For this review, take the finished solid that the model builds, in its own axes (mm). Give positions to 0.01 mm unless a question says otherwise; leave off trailing zeros. Loops run counter-clockwise (first coordinate to the right, second up) from the corner with the lowest first, then second, coordinate; pieces in that order, holes last.
```python
from build123d import *

# Parameters (mm, degrees)
SKETCH_1_R      = 80
SKETCH_1_R_2    = 4
SKETCH_1_R_3    = 1.02
SKETCH_1_R_4    = 6.269952148
EXTRUDE_1_DEPTH = 3


with BuildPart() as part:
    # ｽｹｯﾁ1 → ﾎﾞｽ - 押し出し1 (new body)
    with BuildSketch(Plane(origin=(0, 0, 0), x_dir=(0, 0, -1), z_dir=(1, 0, 0))):
        Circle(SKETCH_1_R)
        Circle(SKETCH_1_R_2, mode=Mode.SUBTRACT)
        with Locations((4.949747468, 4.949747468)):
            Circle(SKETCH_1_R_3, mode=Mode.SUBTRACT)
        with Locations((7, 0)):
            Circle(SKETCH_1_R_3, mode=Mode.SUBTRACT)
        with Locations((4.949747468, -4.949747468)):
            Circle(SKETCH_1_R_3, mode=Mode.SUBTRACT)
        with Locations((0, -7)):
            Circle(SKETCH_1_R_3, mode=Mode.SUBTRACT)
        with Locations((-4.949747468, -4.949747468)):
            Circle(SKETCH_1_R_3, mode=Mode.SUBTRACT)
        with Locations((-7, 0)):
            Circle(SKETCH_1_R_3, mode=Mode.SUBTRACT)
        with Locations((-4.949747468, 4.949747468)):
            Circle(SKETCH_1_R_3, mode=Mode.SUBTRACT)
        with Locations((0, 7)):
            Circle(SKETCH_1_R_3, mode=Mode.SUBTRACT)
        with Locations((-38, 0)):
            Circle(SKETCH_1_R_4, mode=Mode.SUBTRACT)
        with BuildLine():
            Line((-30.755353243, 42.837057437), (35.175005572, 42.837057437))
            ThreePointArc((35.175005572, 42.837057437), (36.589219135, 43.422843874), (37.175005572, 44.837057437))
            Line((37.175005572, 44.837057437), (37.175005572, 45.489077015))
            ThreePointArc((37.175005572, 45.489077015), (36.589219135, 46.903290577), (35.175005572, 47.489077015))
            Line((35.175005572, 47.489077015), (-30.755353243, 47.489077015))
            ThreePointArc((-30.755353243, 47.489077015), (-32.169566806, 46.903290577), (-32.755353243, 45.489077015))
            Line((-32.755353243, 45.489077015), (-32.755353243, 44.837057437))
            ThreePointArc((-32.755353243, 44.837057437), (-32.169566806, 43.422843874), (-30.755353243, 42.837057437))
        make_face(mode=Mode.SUBTRACT)
        with BuildLine():
            Line((37.175005572, -45.489077015), (37.175005572, -44.837057437))
            ThreePointArc((37.175005572, -44.837057437), (36.589219135, -43.422843874), (35.175005572, -42.837057437))
            Line((35.175005572, -42.837057437), (-30.755353243, -42.837057437))
            ThreePointArc((-30.755353243, -42.837057437), (-32.169566806, -43.422843874), (-32.755353243, -44.837057437))
            Line((-32.755353243, -44.837057437), (-32.755353243, -45.489077015))
            ThreePointArc((-32.755353243, -45.489077015), (-32.169566806, -46.903290577), (-30.755353243, -47.489077015))
            Line((-30.755353243, -47.489077015), (35.175005572, -47.489077015))
            ThreePointArc((35.175005572, -47.489077015), (36.589219135, -46.903290577), (37.175005572, -45.489077015))
        make_face(mode=Mode.SUBTRACT)
    extrude(amount=EXTRUDE_1_DEPTH)


solid = part.part
```
Q1. Consider section D-D on z = 56. Give the boundary of the cut face in (x, y).
Answers:
outline: (0, -57.13) - (3, -57.13) - (3, 57.13) - (0, 57.13) - close
Q2. Consider section B-B on z = 38. Give the boundary of the cut face in (x, y), plus the area to 3 significant figures.
Answers:
outline: (0, -70.4) - (3, -70.4) - (3, -6.27) - (0, -6.27) - close; (0, 6.27) - (3, 6.27) - (3, 70.4) - (0, 70.4) - close
area: 385 mm2
Q3. Mouldability with a two-part tool opening along Z and no side actions: class faces 1 (the flat face through (3, 1, -17)), 2 (the cylindrical face through (1.48, -78.1, 17.34)), 3 (the cylindrical face through (1.479, -3.905, 0.867)) as +Z half, -Z half, draft (parallel to the pull), parting line (faces both ways), or undercut.
Answers:
face 1: draft
face 2: parting line
face 3: undercut
Q4. Consider section A-A on x = 1.9. Count the separate pieces of the cut face and the enclosed holes in it, plus the area to 3 significant figures.
Answers:
separate pieces: 1
enclosed holes: 12
area: 19,300 mm2
Q5. Consider section C-C on y = -69.5. Give the boundary of the cut face in (x, z), plus the area to 3 significant figures.
Answers:
outline: (0, -39.62) - (3, -39.62) - (3, 39.62) - (0, 39.62) - close
area: 238 mm2
Q6. For probe 1 along Y at (x, z) = (0.95, 0); probe 2 along Y at (x, z) = (1.3, 7); probe 3 along Y at (x, z) = (2.65, -9), list the stretches that pass through material, from the lowest coordinate up.
Answers:
probe 1: y = -80 to -47.49, -42.84 to -8.02, -5.98 to -4, 4 to 5.98, 8.02 to 42.84, 47.49 to 80
probe 2: y = -79.69 to -47.49, -42.84 to -1.02, 1.02 to 42.84, 47.49 to 79.69
probe 3: y = -79.49 to -47.49, -42.84 to 42.84, 47.49 to 79.49
Q7. For pin 1 Ø1 at (x, z) = (1.5, -9) entering from +Y; pin 2 Ø0.9 at (x, z) = (2, -13.5) entering from +Y; pin 3 Ø1.5 at (x, z) = (1.5, -15.5) entering from -Y, all flat-tipped, find the tip position at first contact; note any pin that passes through.
Answers:
pin 1: stops at y = 79.55
pin 2: stops at y = 78.93
pin 3: stops at y = -78.63
